Geometry check sheet. Reference: the model listing, model coordinates, mm. A direction names the side the tool comes from. Coordinates: 2 decimals unless noted, no trailing zeros. Order: outer loops, then holes, each group sorted by start corner. A loop starts at its lowest first (then second) coordinate and runs counter-clockwise, first axis right, second up. Notation, with made-up numbers: (-28, 20) - (14, 20) arc R22 ccw to (14, 45) - close; hole circle Ø10 at (-19, 85.5). An arc over 180 degrees is marked (long way). Return JSON: item names as keys, results as strings. Group by question number.
Item 1: Section check D-D on x = -30. Enter the section's corners in (y, z), then the cut area to 3 significant figures.
Item 2: Section check A-A on z = 6. Enter the section's corners in (x, y).
Item 3: Scan lines: probe 1 along X at (y, z) = (-92.5, 6); probe 2 along Y at (x, z) = (0, 4); probe 3 along X at (y, z) = (-72, 4). Record each from-to range of solid material in increasing order.
Item 4: Draft check along X on faces 5 (the flat face through (28, -88, 3)), 6 (the cylindrical face through (6.466, -2.681, 10.479)), 7 (the flat face through (37, -92, 6)). Enter one of: pulls with the +X half, pulls with the -X half, needs draft (parallel to the pull), parting line crosses it, or undercut.
Item 5: Section check C-C on x = 0. Enter the section's corners in (y, z).
Item 6: Tool access check on faces 1 (the cylindrical face through (-14.985, 0.66, 4.437)), 2 (the flat face through (-22, -45, 6)), 3 (the cylindrical face through (0, -88, 6)), 4 (the flat face through (22, -43, 6)). Record the directions out of +Z, -Z, +X, -X, +Y, -Y that give a thin tool (end or side, any length) a straight path to the whole face; none if there is none.
Item 7: Gauge pin test, flat ends, axial feed: pin 1 (1 mm diameter, centred on y = 0, z = 8, fed in from +X); pin 2 (3 mm diameter, centred on x = 24.5, z = 5.5, fed in from +Y); pin 3 (18 mm diameter, centred on x = 0, y = 0, fed in from +Z); pin 4 (1 mm diameter, centred on x = 11.5, z = 5, fed in from +Y). Record the tip position at first contact, or that the pin passes through.
Item 8: Section check B-B on y = -41. Enter the section's corners in (x, z), then the cut area to 3 significant figures.
from build123d import *

# Parameters (mm, degrees)
SKETCH1_R           = 15
SKETCH1_R_2         = 7
BOSS_EXTRUDE2_DEPTH = 12
SKETCH3_R           = 3
CUT_EXTRUDE1_DEPTH  = 125.245724273
SKETCH1_4_R         = 15
SKETCH1_4_R_2       = 7
CUT_EXTRUDE2_DEPTH  = 9
FILLET1_R           = 2


with BuildPart() as part:
    # Sketch1 → Boss-Extrude2 (new body)
    # profile 1 of 2: a face of its own
    with BuildSketch(Plane.XY):
        with BuildLine():
            Line((22, 0), (22, -88))
            Line((22, -88), (37, -88))
            Line((37, -88), (37, -96))
            Line((37, -96), (-37, -96))
            Line((-37, -96), (-37, -88))
            Line((-37, -88), (-22, -88))
            Line((-22, -88), (-22, 0))
            ThreePointArc((-22, 0), (0, 22), (22, 0))
        make_face()
        Circle(SKETCH1_R, mode=Mode.SUBTRACT)
        with BuildLine():
            ThreePointArc((-12, -76), (0, -88), (12, -76))
            Line((12, -76), (12, -32))
            ThreePointArc((12, -32), (0, -20), (-12, -32))
            Line((-12, -32), (-12, -76))
        make_face(mode=Mode.SUBTRACT)
    # profile 2 of 2: a face of its own
    with BuildSketch(Plane.XY):
        Circle(SKETCH1_R)
        Circle(SKETCH1_R_2, mode=Mode.SUBTRACT)
    extrude(amount=BOSS_EXTRUDE2_DEPTH)

    # Sketch3 → Cut-Extrude1 (cut, through all)
    with BuildSketch(Plane.XZ.offset(96)):
        with Locations(Location((-30, 6, 0), (0, 0, 270))):
            Circle(SKETCH3_R)
        with Locations(Location((30, 6, 0), (0, 0, 270))):
            Circle(SKETCH3_R)
    extrude(amount=-CUT_EXTRUDE1_DEPTH, mode=Mode.SUBTRACT)

    # Sketch1_4 → Cut-Extrude2 (cut)
    with BuildSketch(Plane.XY):
        Circle(SKETCH1_4_R)
        Circle(SKETCH1_4_R_2, mode=Mode.SUBTRACT)
    extrude(amount=CUT_EXTRUDE2_DEPTH, mode=Mode.SUBTRACT)

    # Fillet1
    fillet1_edges = [part.edges().sort_by_distance(p)[0] for p in [
        (37, -92, 0),
        (-37, -92, 0),
        (-37, -92, 12),
        (37, -92, 12),
    ]]
    fillet(fillet1_edges, radius=FILLET1_R)


solid = part.part
Computed:
{
 "1": {"outline": "(-96, 0) - (-88, 0) - (-88, 3) - (-96, 3) - close; (-96, 9) - (-88, 9) - (-88, 12) - (-96, 12) - close", "area": "48.0 mm²"},
 "2": {"outline": "(-37, -96) - (-33, -96) - (-33, -88) - (-37, -88) - close; (-27, -96) - (27, -96) - (27, -88) - (22, -88) - (22, 0) arc R22 ccw to (-22, 0) - (-22, -88) - (-27, -88) - close; (33, -96) - (37, -96) - (37, -88) - (33, -88) - close; hole circle Ø30 at (0, 0); hole (-12, -76) arc R12 ccw to (12, -76) - (12, -32) arc R12 ccw to (-12, -32) - close"},
 "3": {"probe 1": "x = -37 to -33, -27 to 27, 33 to 37", "probe 2": "y = -96 to -88, -20 to -15, 15 to 22", "probe 3": "x = -22 to -12, 12 to 22"},
 "4": {"face 5": "needs draft", "face 6": "undercut", "face 7": "pulls with the +X half"},
 "5": {"outline": "(-96, 0) - (-88, 0) - (-88, 12) - (-96, 12) - close; (-20, 0) - (-15, 0) - (-15, 9) - (-7, 9) - (-7, 12) - (-20, 12) - close; (7, 9) - (15, 9) - (15, 0) - (22, 0) - (22, 12) - (7, 12) - close"},
 "6": {"face 1": "-Z", "face 2": "+Z, -Z, -X, +Y", "face 3": "+Z, -Z", "face 4": "+Z, -Z, +X, +Y"},
 "7": {"pin 1": "stops at x = 22", "pin 2": "stops at y = -88", "pin 3": "stops at z = 12", "pin 4": "stops at y = 19.05"},
 "8": {"outline": "(-22, 0) - (-12, 0) - (-12, 12) - (-22, 12) - close; (12, 0) - (22, 0) - (22, 12) - (12, 12) - close", "area": "240 mm²"}
}
